Part model, mm, in its own coordinate system. Face numbers are marked on the shaded views. A direction names the side the tool comes from. Round coordinates to 2 decimals unless told otherwise and drop trailing zeros. Loops run counter-clockwise (first coordinate to the right, second up) from the corner with the lowest first, then second, coordinate; pieces in that order, holes last.
from build123d import *

# Parameters (mm, degrees)
BOSS_EXTRUDE1_DEPTH  = 42
FILLET1_R            = 2
BOSS_EXTRUDE2_DEPTH  = 9
FILLET2_R            = 2
CUT_EXTRUDE1_DEPTH   = 9
FILLET3_R            = 2
FILLET2_OF_MIRROR3_R = 2
FILLET3_OF_MIRROR3_R = 2
SKETCH5_R            = 1.5
CUT_EXTRUDE2_DEPTH   = 9
SKETCH7_R            = 2.5
CUT_EXTRUDE3_DEPTH   = 9
SKETCH8_R            = 2.5
CUT_EXTRUDE4_DEPTH   = 9
SKETCH9_R            = 4
SKETCH9_R_2          = 1.5
CUT_EXTRUDE5_DEPTH   = 9
SKETCH10_R           = 1.5
SKETCH10_R_2         = 4
CUT_EXTRUDE6_DEPTH   = 9


with BuildPart() as part:
    # Sketch2 → Boss-Extrude1 (new body)
    with BuildSketch(Plane.XY):
        with BuildLine():
            ThreePointArc((0, 1.792201759), (0.553343721, 0.553343721), (1.792201759, 0))
            Line((1.792201759, 0), (2, 0))
            Line((2, 0), (36, 0))
            Line((36, 0), (36, 1.792224077))
            Line((36, 1.792224077), (2.665691545, 1.792224077))
            ThreePointArc((2.665691545, 1.792224077), (2.206352155, 1.99856094), (2, 2.45789346))
            Line((2, 2.45789346), (2, 25))
            Line((2, 25), (0, 25))
            Line((0, 25), (0, 1.792201759))
        make_face()
    extrude(amount=BOSS_EXTRUDE1_DEPTH)

    # Fillet1
    fillet1_edges = [part.edges().sort_by_distance(p)[0] for p in [
        (1, 25, 0),
        (1, 25, 42),
        (36, 0.896112038, 42),
        (36, 0.896112038, 0),
    ]]
    fillet(fillet1_edges, radius=FILLET1_R)

    # Sketch3 → Boss-Extrude2 (add)
    with BuildSketch(Plane(origin=(0, 0, 0), x_dir=(-1, 0, 0), z_dir=(0, 0, -1))):
        with BuildLine():
            Line((-32, 1.792224077), (-29.505638958, 1.792224077))
            ThreePointArc((-29.505638958, 1.792224077), (-29.847420209, 1.944803868), (-30, 2.286585119))
            Line((-30, 2.286585119), (-30, 24))
            Line((-30, 24), (-32, 24))
            Line((-32, 24), (-32, 1.792224077))
        make_face()
        with BuildLine():
            Line((-8, 0), (-8, 1.792224077))
            Line((-8, 1.792224077), (-29.505638958, 1.792224077))
            Line((-29.505638958, 1.792224077), (-32, 1.792224077))
            ThreePointArc((-32, 1.792224077), (-31.446652567, 0.553347433), (-30.207775923, 0))
            Line((-30.207775923, 0), (-30, 0))
            Line((-30, 0), (-8, 0))
        make_face()
    boss_extrude2 = extrude(amount=BOSS_EXTRUDE2_DEPTH)

    # Fillet2
    fillet2_edges = [part.edges().sort_by_distance(p)[0] for p in [
        (8, 0.896112038, -9),
        (31, 24, -9),
        (31, 24, 0),
    ]]
    fillet(fillet2_edges, radius=FILLET2_R)

    # Sketch4 → Cut-Extrude1 (cut)
    with BuildSketch(Plane(origin=(0, 1.792224077, 0), x_dir=(1, 0, 0), z_dir=(0, 1, 0))):
        with BuildLine():
            Line((28.075602478, 0), (28.075602478, -1.97807902))
            Line((28.075602478, -1.97807902), (36, -2))
            ThreePointArc((36, -2), (35.415834928, -0.584165072), (34, 0))
            Line((34, 0), (28.075602478, 0))
        make_face()
    cut_extrude1 = extrude(amount=-CUT_EXTRUDE1_DEPTH, mode=Mode.SUBTRACT)

    # Fillet3
    fillet3_edges = [part.edges().sort_by_distance(p)[0] for p in [
        (36, 0.896112038, 2),
    ]]
    fillet(fillet3_edges, radius=FILLET3_R)

    # Mirror3: Boss-Extrude2, Cut-Extrude1 across plane
    add(boss_extrude2.mirror(Plane(origin=(0, 0, 21), x_dir=(1, 0, 0), z_dir=(0, 0, -1))))
    add(cut_extrude1.mirror(Plane(origin=(0, 0, 21), x_dir=(1, 0, 0), z_dir=(0, 0, -1))), mode=Mode.SUBTRACT)

    # Fillet2 of Mirror3
    fillet2_of_mirror3_edges = [part.edges().sort_by_distance(p)[0] for p in [
        (8, 0.896112038, 51),
        (31, 24, 51),
        (31, 24, 42),
    ]]
    fillet(fillet2_of_mirror3_edges, radius=FILLET2_OF_MIRROR3_R)

    # Fillet3 of Mirror3
    fillet3_of_mirror3_edges = [part.edges().sort_by_distance(p)[0] for p in [
        (36, 0.896112038, 40),
    ]]
    fillet(fillet3_of_mirror3_edges, radius=FILLET3_OF_MIRROR3_R)

    # Sketch5 → Cut-Extrude2 (cut)
    with BuildSketch(Plane.ZY):
        with Locations((39, 12.396100879)):
            Circle(SKETCH5_R)
        with Locations((31.8, 12.396100879)):
            Circle(SKETCH5_R)
        with Locations((24.6, 12.396100879)):
            Circle(SKETCH5_R)
        with Locations((17.4, 12.396100879)):
            Circle(SKETCH5_R)
        with Locations((10.2, 12.396100879)):
            Circle(SKETCH5_R)
        with Locations((3, 12.396100879)):
            Circle(SKETCH5_R)
        with Locations((31.8, 19.596100879)):
            Circle(SKETCH5_R)
        with Locations((31.8, 5.196100879)):
            Circle(SKETCH5_R)
        with Locations((10.2, 19.596100879)):
            Circle(SKETCH5_R)
        with Locations((10.2, 5.196100879)):
            Circle(SKETCH5_R)
    extrude(amount=-CUT_EXTRUDE2_DEPTH, mode=Mode.SUBTRACT)

    # Sketch7 → Cut-Extrude3 (cut)
    with BuildSketch(Plane(origin=(0, 1.792224077, 0), x_dir=(1, 0, 0), z_dir=(0, 1, 0))):
        with Locations(Location((25.217307954, -46.754456755, 0), (0, 0, 270))):
            Circle(SKETCH7_R)
        with Locations(Location((13.806043378, -46.754456755, 0), (0, 0, 270))):
            Circle(SKETCH7_R)
    cut_extrude3 = extrude(amount=-CUT_EXTRUDE3_DEPTH, mode=Mode.SUBTRACT)

    # Mirror4: Cut-Extrude3 across plane
    add(cut_extrude3.mirror(Plane(origin=(0, 0, 21), x_dir=(1, 0, 0), z_dir=(0, 0, -1))), mode=Mode.SUBTRACT)

    # Sketch8 → Cut-Extrude4 (cut)
    with BuildSketch(Plane.ZY.offset(-30)):
        with Locations((46.754456755, 18.460059087)):
            Circle(SKETCH8_R)
        with Locations((46.754456755, 8.801060864)):
            Circle(SKETCH8_R)
    cut_extrude4 = extrude(amount=-CUT_EXTRUDE4_DEPTH, mode=Mode.SUBTRACT)

    # Mirror5: Cut-Extrude4 across plane
    add(cut_extrude4.mirror(Plane(origin=(0, 0, 21), x_dir=(1, 0, 0), z_dir=(0, 0, -1))), mode=Mode.SUBTRACT)

    # Sketch9 → Cut-Extrude5 (cut)
    with BuildSketch(Plane(origin=(0, 1.792224077, 0), x_dir=(1, 0, 0), z_dir=(0, 1, 0))):
        with Locations(Location((25.217307954, -9.245543245, 0), (0, 0, 270))):
            Circle(SKETCH9_R)
        with Locations(Location((25.217307954, -2.245543245, 0), (0, 0, 270))):
            Circle(SKETCH9_R_2)
        with Locations(Location((32.217307954, -9.245543245, 0), (0, 0, 270))):
            Circle(SKETCH9_R_2)
        with Locations(Location((25.217307954, -16.245543245, 0), (0, 0, 270))):
            Circle(SKETCH9_R_2)
        with Locations(Location((18.217307954, -9.245543245, 0), (0, 0, 270))):
            Circle(SKETCH9_R_2)
    cut_extrude5 = extrude(amount=-CUT_EXTRUDE5_DEPTH, mode=Mode.SUBTRACT)

    # Mirror6: Cut-Extrude5 across plane
    add(cut_extrude5.mirror(Plane(origin=(0, 0, 21), x_dir=(1, 0, 0), z_dir=(0, 0, -1))), mode=Mode.SUBTRACT)

    # Sketch10 → Cut-Extrude6 (cut)
    with BuildSketch(Plane(origin=(0, 1.792224077, 0), x_dir=(1, 0, 0), z_dir=(0, 1, 0))):
        with BuildLine():
            ThreePointArc((15.306043378, -13.341463842), (14.86670355, -12.28080367), (13.806043378, -11.841463842))
            Line((13.806043378, -11.841463842), (13.806043378, -14.841463842))
            ThreePointArc((13.806043378, -14.841463842), (14.86670355, -14.402124014), (15.306043378, -13.341463842))
        make_face()
        with BuildLine():
            Line((13.806043378, -14.841463842), (13.806043378, -11.841463842))
            ThreePointArc((13.806043378, -11.841463842), (12.306043378, -13.341463842), (13.806043378, -14.841463842))
        make_face()
        with Locations(Location((6.901963975, -20.245543245, 0), (0, 0, 270))):
            Circle(SKETCH10_R)
        with Locations(Location((20.710122781, -20.245543245, 0), (0, 0, 270))):
            Circle(SKETCH10_R)
        with Locations(Location((13.806043378, -27.149622647, 0), (0, 0, 270))):
            Circle(SKETCH10_R)
        with Locations(Location((13.806043378, -20.245543245, 0), (0, 0, 270))):
            Circle(SKETCH10_R_2)
    extrude(amount=-CUT_EXTRUDE6_DEPTH, mode=Mode.SUBTRACT)


solid = part.part
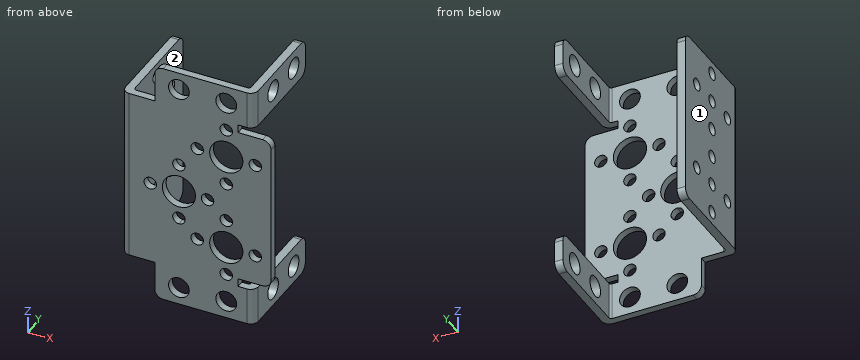
1) Slice it at A-A, the plane y = 15.25. Give the cut face in (x, z), then the cut area to 3 significant figures.
Values:
outline: (0, 0) - (2, 0) - (2, 42) - (0, 42) - close; (30, -9) - (32, -9) - (32, 0) - (30, 0) - close; (30, 42) - (32, 42) - (32, 51) - (30, 51) - close
area: 120 mm2
2) Wall check: line 1 along Y through (x, z) = (15.5, 5); line 2 along X through (y, z) = (15, 47.5); line 3 along X through (y, z) = (3, 40). Give the ranges that are in metal, low to high.
Values:
line 1: y = 0 to 1.79
line 2: x = 30 to 32
line 3: x = 0 to 2
3) Slice it at B-B, the plane z = 3. Give the cut face in (x, y), then the cut area to 3 significant figures.
Values:
outline: (0, 1.79) arc R1.9 ccw to (1.79, 0) - (23.92, 0) - (23.92, 1.79) - (2.67, 1.79) arc R0.71 cw to (2, 2.46) - (2, 10.9) - (0, 10.9) - close; (0, 13.9) - (2, 13.9) - (2, 25) - (0, 25) - close; (26.51, 0) - (35.74, 0) - (35.74, 1.79) - (26.51, 1.79) - close
area: 99.2 mm2
4) Slice it at C-C, the plane z = 10. Give the number of separate pieces and of enclosed holes in the cut face, then the cut area to 3 significant figures.
Values:
separate pieces: 7
enclosed holes: 0
area: 69.1 mm2
5) Tool access for the marked faces 1 and 2: list every direction of +Z, -Z, +X, -X, +Y, -Y with a clear straight run to the whole face (end or side of a thin tool).
Values:
face 1: +Z, -Z, -X, +Y, -Y
face 2: +Z, -Z, +X, +Y
6) Drop flat-ended pins along their axis: pin 1 Ø10 at (x, z) = (17, 29.5) entering from +Y; pin 2 Ø2.5 at (y, z) = (12.4, 31.8) entering from -X; pin 3 Ø1.4 at (y, z) = (1, -2.5) entering from -X; pin 4 Ø7 at (y, z) = (11, -5) entering from +X. Give the stop position or say it passes through.
Values:
pin 1: stops at y = 1.79
pin 2: passes through
pin 3: stops at x = 8
pin 4: stops at x = 32
